Can you work these out from the model? Positions are in its coordinate system, mm. A direction names the side the tool comes from. Round coordinates to 2 decimals unless told otherwise and drop trailing zeros. Write each loop counter-clockwise with the first axis right and the second up, starting at its lowest first coordinate (ties: lowest second). Pieces come first, ordered by that corner, then holes. Notation, with made-up numbers: (29, -14.5) - (38, -14.5) arc R26 cw to (38, 18.5) - close; hole circle Ø7 at (-31, 85.25). An arc over 180 degrees is marked (long way). One line per item, written item: value. Start each with the question number.
(1) Thinking about a two-plate mould opening in Z: for faces 1 (the face through (-92.985, 6.261, -20.648)), 2 (the face through (64, 0, -29)), 3 (the face through (-1.707, 6.439, -79.873)), 4 (the face through (-55.2, 6.4, -58.5)), which applies, +Z half, -Z half, draft (parallel to the pull), parting line (faces both ways), or undercut?
(2) On a 3-axis mill with a long thin cutter (end or side, diameter ignored), from which of +Z, -Z, +X, -X, +Y, -Y can I reach the whole of each face in a straight line? I mean faces 5 (the face through (58.5, 6.4, -55.2)), 6 (the face through (56, 3.861, 36)). Say none if no direction works.
(3) I want a section at D-D on x = 82.55. List the corners of the cut face in (y, z) for me (3 decimals), plus the area to 3 significant figures.
(4) I want a section at C-C on z = 82.55. List the corners of the cut face in (x, y) for me (3 decimals).
(5) If I drill on L1, parallel to Y at x = 30, z = -17; L2, parallel to Z at x = -42, y = 1.5; L3, parallel to Z at x = 55.5, y = 6.25, over which ranges is the centre line in solid material (lowest first)? Write a range as from..to.
(6) I want a section at A-A on z = 0. Give the number of separate pieces and of enclosed holes in the cut face, plus the area to 3 significant figures.
(7) I'm going to push flat-ended pins straight in: pin 1 Ø5.5 at (x, z) = (-82.55, 0) entering from +Y; pin 2 Ø6 at (y, z) = (11, -25) entering from -X; pin 3 Ø1.5 at (x, z) = (-26, -47) entering from -Y; pin 4 Ø1.5 at (y, z) = (9.5, 4) entering from +X. Where does each tip first touch, or does it pass through?
from build123d import *

# Parameters (mm, degrees)
SKETCH1_R                        = 95.25
BOSS_EXTRUDE1_DEPTH              = 12.7
F_1_4_0_25_DIAMETER_HOLE1_D      = 6.35
CIRPATTERN1_COUNT                = 8
SKETCH7_R                        = 69.9135
CUT_EXTRUDE3_DEPTH               = 2.54
SKETCH2_R                        = 68.3133
SKETCH2_R_2                      = 66.1289
CUT_EXTRUDE1_DEPTH               = 1.3208
F_45_64_0_70313_DIAMETER_HOLE1_D = 17.859502


with BuildPart() as part:
    # Sketch1 → Boss-Extrude1 (new body)
    with BuildSketch(Plane(origin=(0, 0, 0), x_dir=(1, 0, 0), z_dir=(0, 1, 0))):
        with Locations(Location((0, 0, 0), (0, 0, 270))):
            Circle(SKETCH1_R)
    extrude(amount=BOSS_EXTRUDE1_DEPTH)

    # 1/4 (0.25) Diameter Hole1 (through all)
    with Locations(Plane(origin=(0, 0, 0), x_dir=(-1, 0, 0), z_dir=(0, -1, 0))):
        with Locations((0, -82.55)):
            f_1_4_0_25_diameter_hole1 = Hole(F_1_4_0_25_DIAMETER_HOLE1_D / 2)

    # CirPattern1: 1/4 (0.25) Diameter Hole1 ×8 about axis
    cirpattern1_axis = Axis((0, 0, 0), (0, 1, 0))
    for i in range(1, CIRPATTERN1_COUNT):
        add(f_1_4_0_25_diameter_hole1.rotate(cirpattern1_axis, i * 360 / CIRPATTERN1_COUNT), mode=Mode.SUBTRACT)

    # Sketch7 → Cut-Extrude3 (cut)
    with BuildSketch(Plane(origin=(0, 0, 0), x_dir=(-1, 0, 0), z_dir=(0, -1, 0))):
        with Locations(Location((0, 0, 0), (0, 0, 90))):
            Circle(SKETCH7_R)
    extrude(amount=-CUT_EXTRUDE3_DEPTH, mode=Mode.SUBTRACT)

    # Sketch2 → Cut-Extrude1 (cut)
    with BuildSketch(Plane.XZ.offset(-2.54)):
        with Locations(Location((0, 0, 0), (0, 0, 270))):
            Circle(SKETCH2_R)
        with Locations(Location((0, 0, 0), (0, 0, 270))):
            Circle(SKETCH2_R_2, mode=Mode.SUBTRACT)
    extrude(amount=-CUT_EXTRUDE1_DEPTH, mode=Mode.SUBTRACT)

    # 45/64 (0.70313) Diameter Hole1 (through all)
    with Locations(Plane(origin=(0, 2.54, 0), x_dir=(-1, 0, 0), z_dir=(0, -1, 0))):
        with Locations((0, 0)):
            Hole(F_45_64_0_70313_DIAMETER_HOLE1_D / 2)


solid = part.part
Established:
1. face 1: parting line
1. face 2: draft
1. face 3: undercut
1. face 4: undercut
2. face 5: +Y, -Y
2. face 6: -Y
3. outline: (0, -47.519) - (12.7, -47.519) - (12.7, -3.175) - (0, -3.175) - close; (0, 3.175) - (12.7, 3.175) - (12.7, 47.519) - (0, 47.519) - close
3. area: 1,130 mm2
4. outline: (-47.519, 0) - (-3.175, 0) - (-3.175, 12.7) - (-47.519, 12.7) - close; (3.175, 0) - (47.519, 0) - (47.519, 12.7) - (3.175, 12.7) - close
5. L1: 2.54..12.7
5. L2: -85.49..-55.89, 55.89..85.49
5. L3: -77.41..-59.73, -57.02..57.02, 59.73..77.41
6. separate pieces: 4
6. enclosed holes: 0
6. area: 1,720 mm2
7. pin 1: through
7. pin 2: x = -92.67
7. pin 3: y = 2.54
7. pin 4: x = 95.19
